```python
from build123d import *

# Parameters (mm, degrees)
F1_DEPTH = 25.4


with BuildPart() as f1:
    # F0 (on Top) → F1 (new body)
    with BuildSketch(Plane.XY):
        with BuildLine():
            ThreePointArc((-59.1107523799, 49.5368446501), (-61.6481766526, 46.5452847002), (-60.2000903929, 42.8996024515))
            Line((-60.2000903929, 42.8996024515), (-47.3238480687, 33.0717364155))
            Line((-47.3238480687, 33.0717364155), (-38.8923999974, 35.9275490176))
            ThreePointArc((-38.8923999974, 35.9275490176), (-38.5200626671, 38.7717193747), (-36.1004724001, 37.2310951352))
            ThreePointArc((-36.1004724001, 37.2310951352), (-36.1107927824, 37.0440430671), (-36.1416286435, 36.8592617474))
            Line((-36.1416286435, 36.8592617474), (-19.4805414172, 42.5025323296))
            Line((-19.4805414172, 42.5025323296), (-24.4742741518, 57.2459360816))
            ThreePointArc((-24.4742741518, 57.2459360816), (-26.3954934154, 59.4396204364), (-29.3051696679, 59.6322823499))
            Line((-29.3051696679, 59.6322823499), (-59.1107523799, 49.5368446501))
        make_face()
        with BuildLine():
            Line((-38.8923999974, 35.9275490176), (-47.3238480687, 33.0717364155))
            Line((-47.3238480687, 33.0717364155), (-42.6756189918, 29.5239488295))
            Line((-42.6756189918, 29.5239488295), (-17.9241616526, 37.907505627))
            Line((-17.9241616526, 37.907505627), (-19.4805414172, 42.5025323296))
            Line((-19.4805414172, 42.5025323296), (-36.1416286435, 36.8592617474))
            ThreePointArc((-36.1416286435, 36.8592617474), (-37.2552876391, 35.6206883909), (-38.8923999974, 35.9275490176))
        make_face()
        with BuildLine():
            Line((-17.9241616526, 37.907505627), (-42.6756189918, 29.5239488295))
            Line((-42.6756189918, 29.5239488295), (-36.3345149505, 24.6840646871))
            Line((-36.3345149505, 24.6840646871), (-41.3134286256, 5.9786473972))
            ThreePointArc((-41.3134286256, 5.9786473972), (-36.7132008564, 2.606335405), (-31.6395828713, 0))
            ThreePointArc((-31.6395828713, 0), (-12.0320170539, -2.3394482542), (5.8771688615, 5.9786473972))
            Line((5.8771688615, 5.9786473972), (19.1956014543, 0.00967121))
            ThreePointArc((19.1956014543, 0.00967121), (34.4581492923, 18.4761157552), (49.587438224, 37.0518945294))
            Line((49.587438224, 37.0518945294), (41.8655847635, 41.4393103907))
            Line((41.8655847635, 41.4393103907), (38.9125214018, 43.117186965))
            Line((38.9125214018, 43.1171869651), (41.8593864064, 47.2519499851))
            Line((41.8593864064, 47.2519499851), (14.8451968214, 22.2191433988))
            ThreePointArc((14.8451968214, 22.2191433988), (1.1174172166, 12.3750160433), (-12.6103623883, 22.2191433988))
            Line((-12.6103623883, 22.2191433988), (-17.9241616526, 37.907505627))
        make_face()
        with BuildLine():
            ThreePointArc((-31.6395828713, 0), (-36.7132008564, 2.606335405), (-41.3134286256, 5.9786473972))
            Line((-41.3134286256, 5.9786473972), (-44.7103866945, 0))
            Line((-44.7103866945, 0), (-44.7103866945, -32.1961882046))
            ThreePointArc((-44.7103866945, -32.1961882046), (-35.6981979706, -34.6212321144), (-26.8360574654, -37.5474667641))
            ThreePointArc((-26.8360574654, -37.5474667641), (-20.5610394294, -34.4552816286), (-14.112735744, -31.7429321219))
            ThreePointArc((-14.112735744, -31.7429321219), (-22.7734524474, -28.9208943273), (-31.6395828713, -26.8319610022))
            Line((-31.6395828713, -26.8319610022), (-31.6395828713, 0))
        make_face()
        with BuildLine():
            Line((19.1956014543, 0.00967121), (5.8771688615, 5.9786473972))
            Line((5.8771688615, 5.9786473972), (5.8771688615, -26.0057745091))
            ThreePointArc((5.8771688615, -26.0057745091), (-4.2452726756, -28.4301442134), (-14.112735744, -31.7429321219))
            ThreePointArc((-14.112735744, -31.7429321219), (-7.332536937, -34.533476308), (-0.7553169871, -37.7736013745))
            ThreePointArc((-0.7553169871, -37.7736013745), (9.143147591, -34.2583484987), (19.1956014543, -31.2112556035))
            Line((19.1956014543, -31.2112556035), (19.1956014543, 0.00967121))
        make_face()
        Polygon((41.9694184521, 47.4456064242), (41.8593864064, 47.2519499851), (38.9125214018, 43.1171869651), (41.8655847635, 41.4393103907), (45.162112145, 45.4186524008), align=None)
        with BuildLine():
            ThreePointArc((-0.7553169871, -37.7736013745), (-7.332536937, -34.533476308), (-14.112735744, -31.7429321219))
            ThreePointArc((-14.112735744, -31.7429321219), (-20.5610394294, -34.4552816286), (-26.8360574654, -37.5474667641))
            ThreePointArc((-26.8360574654, -37.5474667641), (-20.074389371, -40.1601770998), (-13.4328625364, -43.064747984))
            ThreePointArc((-13.4328625364, -43.064747984), (-7.1346825518, -40.3219146743), (-0.7553169871, -37.7736013745))
        make_face()
        with BuildLine():
            ThreePointArc((-13.4328625364, -43.064747984), (-20.074389371, -40.1601770998), (-26.8360574654, -37.5474667641))
            ThreePointArc((-26.8360574654, -37.5474667641), (-37.8079228806, -44.1596970981), (-47.9927124606, -51.9297345425))
            ThreePointArc((-47.9927124606, -51.9297345425), (-55.1060167541, -64.9103960311), (-47.7461889386, -77.7528882027))
            ThreePointArc((-47.7461889386, -77.7528882027), (-12.4874489881, -79.2604436558), (22.7598436177, -77.5054991245))
            ThreePointArc((22.7598436177, -77.5054991245), (25.753425112, -65.9683634877), (22.5124526769, -54.4982664287))
            ThreePointArc((22.5124526769, -54.4982664287), (11.4306480238, -45.3678662365), (-0.7553169871, -37.7736013745))
            ThreePointArc((-0.7553169871, -37.7736013745), (-7.1346825518, -40.3219146743), (-13.4328625364, -43.064747984))
        make_face()
        with BuildLine():
            ThreePointArc((-38.401431896, -56.3598381515), (-26.127337959, -49.3175486866), (-13.4328625364, -43.064747984))
            ThreePointArc((-13.4328625364, -43.064747984), (-1.1655138535, -49.3811780371), (10.536660869, -56.691734725))
            ThreePointArc((10.536660869, -56.691734725), (13.6866926882, -61.5483388363), (14.1682401614, -67.3169969113))
            ThreePointArc((14.1682401614, -67.3169969113), (-12.073405036, -69.8014865929), (-38.401431896, -68.5241325674))
            ThreePointArc((-38.401431896, -68.5241325674), (-40.6616602948, -62.4419853594), (-38.401431896, -56.3598381515))
        make_face(mode=Mode.SUBTRACT)
        with BuildLine():
            ThreePointArc((47.1642236558, 48.8760605112), (44.2705643123, 49.2367128523), (41.9694184521, 47.4456064242))
            Line((41.9694184521, 47.4456064242), (45.162112145, 45.4186524008))
            Line((45.162112145, 45.4186524008), (52.5536226058, 40.7259842943))
            ThreePointArc((52.5536226058, 40.7259842943), (53.3304416036, 43.828541799), (51.4696137823, 46.4298166105))
            Line((51.4696137823, 46.4298166105), (47.1642236558, 48.8760605112))
        make_face()
        with BuildLine():
            Line((41.8655847635, 41.4393103907), (49.587438224, 37.0518945294))
            ThreePointArc((49.587438224, 37.0518945294), (51.0711817018, 38.8884136117), (52.5536226058, 40.7259842943))
            Line((52.5536226058, 40.7259842943), (45.162112145, 45.4186524008))
            Line((45.162112145, 45.4186524008), (41.8655847635, 41.4393103907))
        make_face()
    extrude(amount=F1_DEPTH)


solid = f1.part
```
Source: CAD feature listing. Evaluate the final solid. Frame: model axes, mm. A direction names the side the tool comes from. Give positions to 0.01 mm unless a question says otherwise; leave off trailing zeros. Write each loop counter-clockwise with the first axis right and the second up, starting at its lowest first coordinate (ties: lowest second). Pieces come first, ordered by that corner, then holes. Notation, with made-up numbers: (61, 44.25) - (116, 44.25) arc R10 cw to (116, 51.25) - close; hole circle Ø5 at (11, 32.25). An arc over 180 degrees is marked (long way). One line per item, written item: value. Start each with the question number.
Q1. Draft query along X for faces 1 (the face through (8, -9, 25.4)), 2 (the face through (-61.64, 46.6, 12.52)), 3 (the face through (-26.3, -49.41, 12.52)). Return one class per face: +X half, -X half, draft (parallel to the pull), parting line (faces both ways), or undercut.
Q2. Section query C-C, the plane x = -51.5. Return the cut outline in (y, z), then the cut area to 3 significant figures.
Q3. Section query D-D, the plane z = 11.75. Count the separate pieces of the cut face and the enclosed holes in it, then the cut area to 3 significant figures.
Q4. First-contact query: pin 1 Ø12.5 at (y, z) = (-6, 19) entering from -X; pin 2 Ø2 at (y, z) = (-49, 11) entering from +X; pin 3 Ø10 at (x, z) = (-38, 8.5) entering from +Y. Flat tips, straight axial feed; report the tip coordinate or a pass-through.
Q5. Material intervals for probe 1 along X at (y, z) = (-20, 8.25); probe 2 along Y at (x, z) = (-10, 7.75); probe 3 along Y at (x, z) = (-27.5, 11.75), sorted ascending. Write a range as from..to.
Q6. Section query A-A, the plane x = 3.5. Return the cut outline in (y, z).
Q7. Set-up query: faces 4 (the face through (-11.704, -69.793, 12.522)), 5 (the face through (44.311, 49.248, 12.522)), 6 (the face through (34.25, 18.22, 12.52)), 7 (the face through (-42.99, 3.03, 12.52)). Return all of +Z, -Z, +X, -X, +Y, -Y with unobstructed straight access to the full face (end or side cutting, diameter ignored); none if empty.
Q8. Section query B-B, the plane y = -15.5. Return the cut outline in (x, z), then the cut area to 3 significant figures.
Answer:
1. face 1: draft
1. face 2: -X half
1. face 3: undercut
2. outline: (-74.57, 0) - (-54.96, 0) - (-54.96, 25.4) - (-74.57, 25.4) - close; (36.26, 0) - (52.11, 0) - (52.11, 25.4) - (36.26, 25.4) - close
2. area: 901 mm2
3. separate pieces: 1
3. enclosed holes: 3
3. area: 5,880 mm2
4. pin 1: stops at x = -44.71
4. pin 2: stops at x = 17.42
4. pin 3: stops at y = 58.38
5. probe 1: x = -44.71..-31.64, 5.88..19.2
5. probe 2: y = -79.24..-69.74, -44.7..-30.24, -1.96..17.57
5. probe 3: y = -79.02..-69.51, -50.05..-37.9, -37.31..-27.71, -1.44..59.79
6. outline: (-78.87, 0) - (-68.78, 0) - (-68.78, 25.4) - (-78.87, 25.4) - close; (-52.13, 0) - (-40.18, 0) - (-40.18, 25.4) - (-52.13, 25.4) - close; (-36.2, 0) - (-26.49, 0) - (-26.49, 25.4) - (-36.2, 25.4) - close; (4.1, 0) - (12.57, 0) - (12.57, 25.4) - (4.1, 25.4) - close
7. face 4: +Z, -Z
7. face 5: +Z, -Z, +Y
7. face 6: +Z, -Z, +X
7. face 7: +Z, -Z, -X
8. outline: (-44.71, 0) - (-31.64, 0) - (-31.64, 25.4) - (-44.71, 25.4) - close; (5.88, 0) - (19.2, 0) - (19.2, 25.4) - (5.88, 25.4) - close
8. area: 670 mm2
